Geometry: see drawing. Coordinates: mm, zero at the bounding-box minimum. A direction names the side the tool comes from. Coordinates: 2 decimals unless noted, no trailing zeros. Order: outer loops, then holes, each group sorted by start corner. A loop starts at its lowest first (then second) coordinate and runs counter-clockwise, first axis right, second up. Notation, with made-up numbers: (-19, 55) - (28, 55) arc R28 cw to (28, 80) - close; hole circle Ø6 at (71, -36.75). An arc over 180 degrees is marked (long way). Use a Markdown table: item, result. Add a question column.
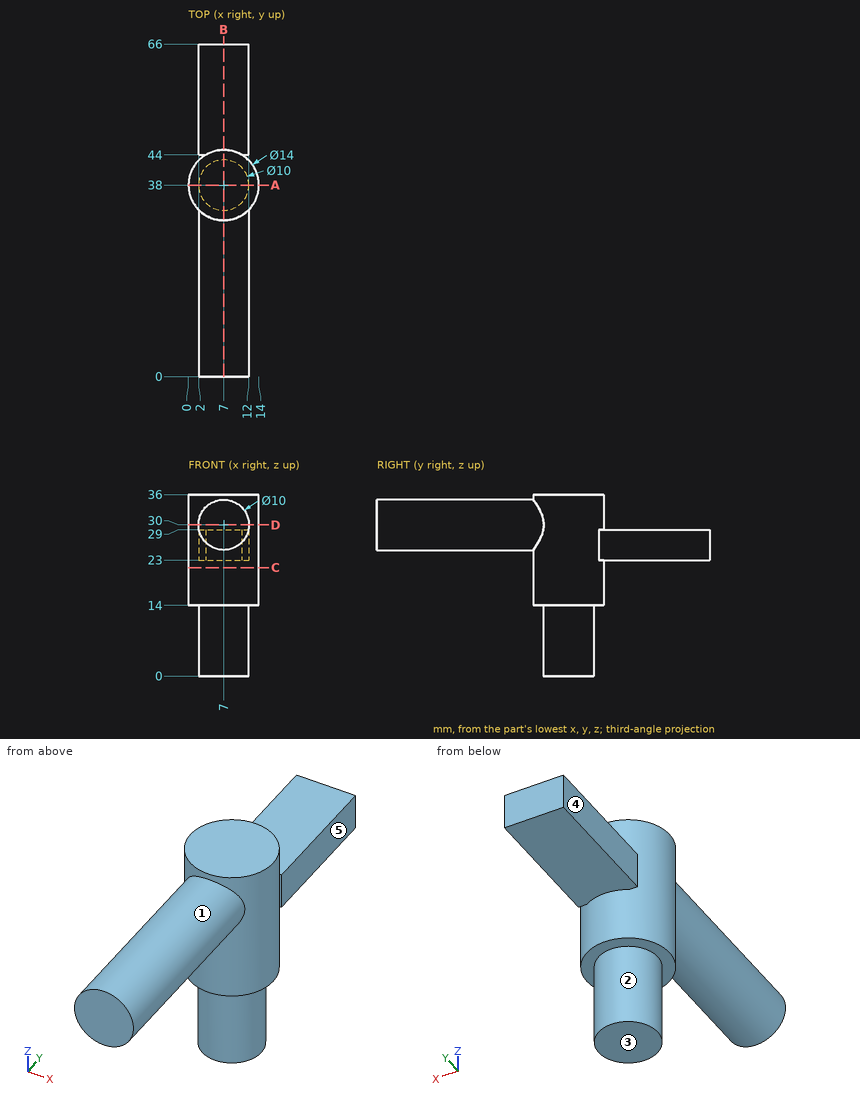
1) Section query D-D (z = 30). Return the cut outline in (x, y), and give its area (3 significant figures).
2) First-contact query: pin 1 (5 mm diameter, centred on x = 9.5, y = 57.5, fed in from -Z); pin 2 (4 mm diameter, centred on x = 2.5, z = 32, fed in from +Y); pin 3 (5 mm diameter, centred on y = 59, z = 27, fed in from -X). Flat tips, straight axial feed; report the tip coordinate or a pass-through.
3) Section query C-C (z = 21.5). Return the cut outline in (x, y).
4) Section query A-A (y = 38). Return the cut outline in (x, z), and give its area (3 significant figures).
5) Section query B-B (x = 7). Return the cut outline in (y, z).
6) Access query for the marked faces 1, 2, 3, 4 and 5. Directions: +Z, -Z, +X, -X, +Y, -Y. A direction counts if a zero-diameter tool reaches every point of the face in a straight line with its end or side. Return the directions, or none.
7) Line query: line 1 (Z direction, x = 9.25, y = 50.5); line 2 (Z direction, x = 1.25, y = 39.5); line 3 (Y direction, x = 2.75, z = 16). Output: solid intervals per line, ascending. Write a range as from..to.
From the geometry:
| question | item | result |
|---|---|---|
| 1 | outline | (2, 0) - (12, 0) - (12, 33.1) arc R7 ccw (long way) to (2, 33.1) - close |
| 1 | area | 470 mm^2 |
| 2 | pin 1 | stops at z = 23 |
| 2 | pin 2 | stops at y = 44.54 |
| 2 | pin 3 | stops at x = 2 |
| 3 | outline | circle Ø14 at (7, 38) |
| 4 | outline | (0, 14) - (2, 14) - (2, 0) - (12, 0) - (12, 14) - (14, 14) - (14, 36) - (0, 36) - close |
| 4 | area | 448 mm^2 |
| 5 | outline | (0, 25) - (31, 25) - (31, 14) - (33, 14) - (33, 0) - (43, 0) - (43, 14) - (45, 14) - (45, 23) - (66, 23) - (66, 29) - (45, 29) - (45, 36) - (31, 36) - (31, 35) - (0, 35) - close |
| 6 | face 1 | -Y |
| 6 | face 2 | -Z |
| 6 | face 3 | -Z, +X, -X, +Y, -Y |
| 6 | face 4 | +Z, -Z, -X, +Y |
| 6 | face 5 | +Z, -Z, +X, +Y |
| 7 | line 1 | z = 23..29 |
| 7 | line 2 | z = 14..36 |
| 7 | line 3 | y = 32.44..43.56 |
